Can you work these out from the drawing? Everything is in mm from the part's minimum corner. Round coordinates to 2 decimals unless told otherwise and drop trailing zeros. Write each loop counter-clockwise with the first axis right and the second up, starting at its lowest first coordinate (ties: lowest second). Pieces come first, ordered by that corner, then holes. Notation, with made-up numbers: (-39, 63.25) - (-8, 63.25) arc R21 ccw to (-8, 86.25) - close; hole circle Ø4 at (39, -24.75). An arc over 180 degrees is marked (long way). One line per item, written item: value. Start each with the question number.
(1) I want a section at A-A on y = 2.5. List the corners of the cut face in (x, z) for me, plus the area to 3 significant figures.
(2) I want a section at B-B on x = 2.5. List the corners of the cut face in (y, z) for me.
(3) I'm going to push a flat-ended pin straight in: pin 1 Ø2 at (x, y) = (55.5, 1.5) entering from -Z. Where does the tip first touch, or does it pass through?
(4) I want a section at C-C on z = 2.1. List the corners of the cut face in (x, y) for me, plus the area to 3 significant figures.
(5) If I drill on L1, parallel to Y at x = 61.8, z = 1; L2, parallel to X at y = 3.8, z = 2; L3, parallel to X at y = 1.45, z = 1.35, over which ranges is the centre line in solid material (lowest first)? Write a range as from..to.
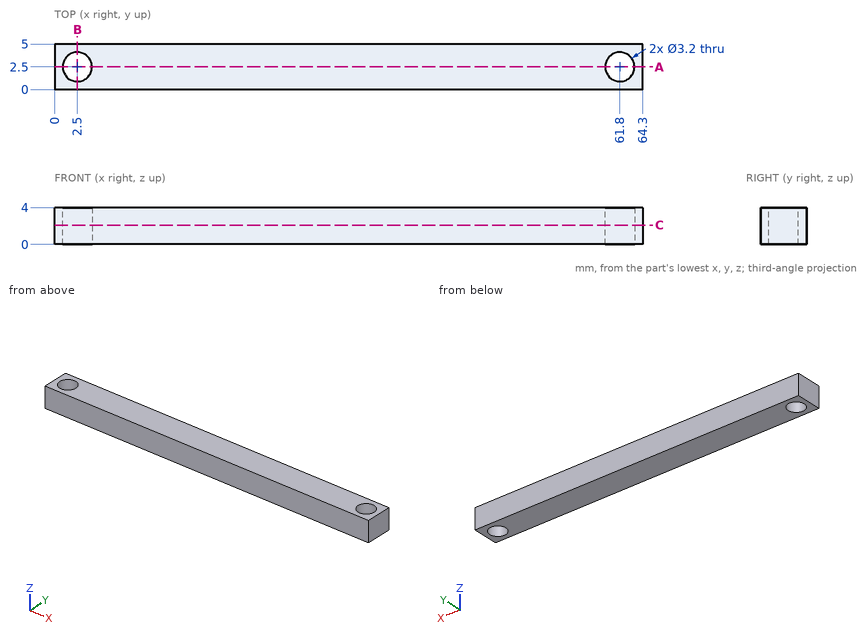
Established:
1. outline: (0, 0) - (0.9, 0) - (0.9, 4) - (0, 4) - close; (4.1, 0) - (60.2, 0) - (60.2, 4) - (4.1, 4) - close; (63.4, 0) - (64.3, 0) - (64.3, 4) - (63.4, 4) - close
1. area: 232 mm2
2. outline: (0, 0) - (0.9, 0) - (0.9, 4) - (0, 4) - close; (4.1, 0) - (5, 0) - (5, 4) - (4.1, 4) - close
3. pin 1: z = 0
4. outline: (0, 0) - (64.3, 0) - (64.3, 5) - (0, 5) - close; hole circle Ø3.2 at (2.5, 2.5); hole circle Ø3.2 at (61.8, 2.5)
4. area: 305 mm2
5. L1: 0..0.9, 4.1..5
5. L2: 0..1.57, 3.43..60.87, 62.73..64.3
5. L3: 0..1.29, 3.71..60.59, 63.01..64.3
